Build history of the part. All positions in model axes, mm. Face numbers are marked on the shaded views. Round coordinates to 2 decimals unless told otherwise and drop trailing zeros. Write each loop counter-clockwise with the first axis right and the second up, starting at its lowest first coordinate (ties: lowest second). Pieces come first, ordered by that corner, then holes. Notation, with made-up numbers: M 49.5,59 L 92.5,59 A29 cw 92.5,92 Z; hole C -38.5,68 d3. An arc over 180 degrees is marked long. One line per item, written item: value. Start each with the question number.
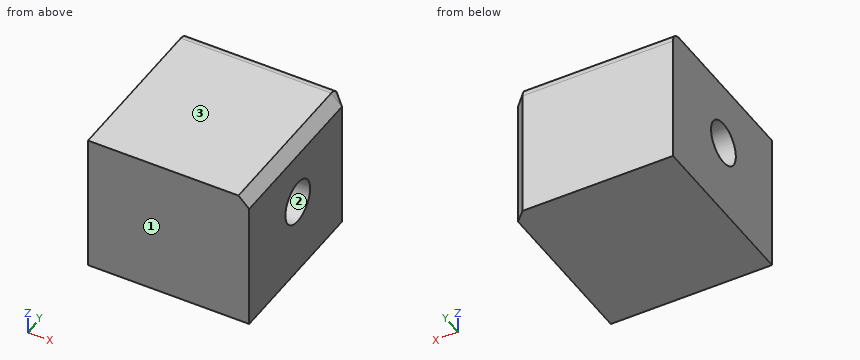
```python
from build123d import *

# Parameters (mm, degrees)
F0_W     = 160
F0_H     = 130
F1_DEPTH = 150
F2_R     = 10
F3_SIZE  = 10
F4_R     = 20
F5_DEPTH = 265


with BuildPart() as f1:
    # F0 (on Right) → F1 (new body)
    with BuildSketch(Plane.YZ):
        with Locations((80, 65)):
            Rectangle(F0_W, F0_H)
    extrude(amount=F1_DEPTH)

    # F2
    f2_edges = [f1.edges().sort_by_distance(p)[0] for p in [
        (75, 160, 130),
    ]]
    fillet(f2_edges, radius=F2_R)

    # F3
    f3_edges = [f1.edges().sort_by_distance(p)[0] for p in [
        (150, 75, 130),
        (150, 160, 60),
        (150, 157.071068, 127.071068),
    ]]
    chamfer(f3_edges, length=F3_SIZE)

    # F4 (on face) → F5 (cut)
    with BuildSketch(Plane.YZ.offset(150)):
        with Locations((78.493013978, 71.4490786195)):
            Circle(F4_R)
    extrude(amount=-F5_DEPTH, mode=Mode.SUBTRACT)


solid = f1.part
```
Item 1: Drop a flat-ended pin along its axis: pin 1 (12 mm diameter, centred on y = 88, z = 62, fed in from +X). Give the stop position or say it passes through.
Item 2: Cut at B-B, the plane x = 81. Write the cut outline in (y, z), plus the area to 3 significant figures.
Item 3: Drill centre lines: line 1 (Z direction, x = 82.5, y = 82); line 2 (Z direction, x = 16.5, y = 63); line 3 (Y direction, x = 18.5, z = 121.5). Where is each one in solid material? Low to high.
Item 4: Two-plate mould, pull along Z, no slides. Class the marked faces 1, 2 and 3: pulls with the +Z half, pulls with the -Z half, needs draft (parallel to the pull), parting line crosses it, or undercut.
Item 5: Cut at A-A, the plane z = 78. Write the cut outline in (x, y).
Computed values:
1. pin 1: passes through
2. outline: M 0,0 L 160,0 L 160,120 A10 ccw 150,130 L 0,130 Z; hole C 78.49,71.45 d40
2. area: 19,500 mm2
3. line 1: z = 0 to 51.76, 91.14 to 130
3. line 2: z = 0 to 58.8, 84.1 to 130
3. line 3: y = 0 to 159.89
4. face 1: needs draft
4. face 2: undercut
4. face 3: pulls with the +Z half
5. outline: M 0,0 L 150,0 L 150,59.6 L 0,59.6 Z; M 0,97.39 L 150,97.39 L 150,150 L 140,160 L 0,160 Z
